from build123d import *

# Parameters (mm, degrees)
F0_W     = 57.9444081523
F0_H     = 26.1267647147
F1_DEPTH = 20
F2_R     = 12.55
F3_R     = 2


with BuildPart() as f1:
    # F0 (on Right) → F1 (new body)
    with BuildSketch(Plane.YZ):
        with Locations((-23.52779801, 31.6725373268)):
            Rectangle(F0_W, F0_H)
    extrude(amount=F1_DEPTH)

    # F2
    f2_edges = [f1.edges().sort_by_distance(p)[0] for p in [
        (20, -23.527798, 18.609155),
        (20, 5.444406, 31.672537),
        (20, -23.527798, 44.73592),
        (20, -52.500002, 31.672537),
    ]]
    fillet(f2_edges, radius=F2_R)

    # F3
    f3_edges = [f1.edges().sort_by_distance(p)[0] for p in [
        (20, -23.527798, 31.159155),
        (17.029365, -48.057916, 23.051241),
        (17.029365, -48.057916, 40.293833),
        (17.029365, 1.00232, 23.051241),
        (17.029365, 1.00232, 40.293833),
    ]]
    fillet(f3_edges, radius=F3_R)


solid = f1.part
Here's how the part is built. I have some questions about the finished solid (model axes, mm). Coordinates: 2 decimals unless noted, no trailing zeros. Loops run counter-clockwise (first coordinate to the right, second up) from the corner with the lowest first, then second, coordinate; pieces in that order, holes last.
1. I need wall thicknesses on L1, parallel to Z at x = 8, y = -9.5; L2, parallel to X at y = -11, z = 20; L3, parallel to Z at x = 13.75, y = -13 (3 decimals). Which ranges of each line are inside material? Lowest first, please.
2. If we mould it in two halves opening along Z, with no side actions, what happens to faces 1 (the flat face through (0, -24, 32)), 2 (the cylindrical face through (16.23, -23.15, 22.19)), 3 (the cylindrical face through (3.78, 4.84, 44.17))? For each: pulls with the +Z half, pulls with the -Z half, needs draft (parallel to the pull), parting line crosses it, or undercut.
3. For P1, Ø6, axis at x = 11, y = -27.5, coming from the +Z side; P2, Ø12, axis at x = 15.5, y = -13, coming from the +Z side; P3, Ø8, axis at x = 12.5, z = 21.5, coming from the -Y side, each with a flat end and sliding along its axis, tell me the tip position at first contact or that it passes through.
4. Imagine slicing it at A-A, the plane y = -21.5. Please give me the cut outline in (x, z), and give its area (3 significant figures).
Taken from the geometry:
1. L1: z = 18.62 to 44.72
1. L2: x = 0 to 13.19
1. L3: z = 20.305 to 43.04
2. face 1: needs draft
2. face 2: pulls with the -Z half
2. face 3: pulls with the +Z half
3. P1: stops at z = 44.72
3. P2: stops at z = 44.57
3. P3: stops at y = -52.46
4. outline: (0, 18.61) - (7.45, 18.61) arc R12.55 ccw to (20, 31.16) - (20, 32.19) arc R12.55 ccw to (7.45, 44.74) - (0, 44.74) - close
4. area: 455 mm2
